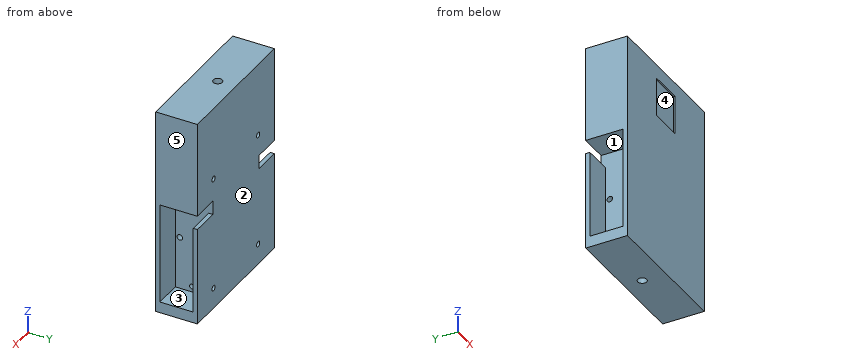
```python
from build123d import *

# Parameters (mm, degrees)
SKETCH1_W                    = 100
SKETCH1_H                    = 150
BOX_DEPTH                    = 30
SKETCH2_W                    = 73
SKETCH2_H                    = 24
MOTOR_COMPARTMENT_DEPTH      = 20
SKETCH3_W                    = 10
SKETCH3_H                    = 3
MOTOR_WIRE_PASSTHROUGH_DEPTH = 20
SKETCH4_R                    = 1.75
SKETCH4_R_2                  = 2
MOTOR_SCREW_MOUNT_DEPTH      = 10
SKETCH5_R                    = 2
MAKER_PI_MOUNT_HOLES_DEPTH   = 8
SKETCH6_W                    = 24
SKETCH6_H                    = 28
CASTER_MOUNT_DEPTH           = 1
SKETCH7_R                    = 3.2
FRONT_MOUNT_HOLE_DEPTH       = 25.4


with BuildPart() as part:
    # Sketch1 → box (new body)
    with BuildSketch(Plane(origin=(0, 0, 0), x_dir=(1, 0, 0), z_dir=(0, 1, 0))):
        Rectangle(SKETCH1_W, SKETCH1_H)
    extrude(amount=-BOX_DEPTH)

    # Sketch2 → motor compartment (cut)
    with BuildSketch(Plane(origin=(50, 0, 0), x_dir=(0, 0, -1), z_dir=(1, 0, 0))):
        with Locations((30.5, -15)):
            Rectangle(SKETCH2_W, SKETCH2_H)
    motor_compartment = extrude(amount=-MOTOR_COMPARTMENT_DEPTH, mode=Mode.SUBTRACT)

    # Sketch3 → motor wire passthrough (cut)
    with BuildSketch(Plane(origin=(50, 0, 0), x_dir=(0, 0, -1), z_dir=(1, 0, 0))):
        with Locations((-1, -1.5)):
            Rectangle(SKETCH3_W, SKETCH3_H)
    motor_wire_passthrough = extrude(amount=-MOTOR_WIRE_PASSTHROUGH_DEPTH, mode=Mode.SUBTRACT)

    # Sketch4 → motor screw mount (cut)
    with BuildSketch(Plane(origin=(30, 0, 0), x_dir=(0, 0, -1), z_dir=(1, 0, 0))):
        with Locations((63, -15)):
            Circle(SKETCH4_R)
        with Locations((28.75, -6.25)):
            Circle(SKETCH4_R_2)
        with Locations(Location((28.75, -23.75, 0), (0, 0, 180))):
            Circle(SKETCH4_R_2)
    motor_screw_mount = extrude(amount=-MOTOR_SCREW_MOUNT_DEPTH, mode=Mode.SUBTRACT)

    # motor compartment mirror: motor compartment, motor wire passthrough, motor screw mount across plane
    add(motor_compartment.mirror(Plane(origin=(0, 0, 0), x_dir=(0, 0, 1), z_dir=(1, 0, 0))), mode=Mode.SUBTRACT)
    add(motor_wire_passthrough.mirror(Plane(origin=(0, 0, 0), x_dir=(0, 0, 1), z_dir=(1, 0, 0))), mode=Mode.SUBTRACT)
    add(motor_screw_mount.mirror(Plane(origin=(0, 0, 0), x_dir=(0, 0, 1), z_dir=(1, 0, 0))), mode=Mode.SUBTRACT)

    # Sketch5 → Maker Pi mount holes (cut)
    with BuildSketch(Plane(origin=(0, 0, 0), x_dir=(1, 0, 0), z_dir=(0, 1, 0))):
        with Locations(Location((-29, 60, 0), (0, 0, 270))):
            Circle(SKETCH5_R)
        with Locations(Location((-29, -22, 0), (0, 0, 270))):
            Circle(SKETCH5_R)
        with Locations(Location((29, 60, 0), (0, 0, 300))):
            Circle(SKETCH5_R)
        with Locations(Location((29, -22, 0), (0, 0, 90))):
            Circle(SKETCH5_R)
    extrude(amount=-MAKER_PI_MOUNT_HOLES_DEPTH, mode=Mode.SUBTRACT)

    # Sketch6 → caster mount (cut)
    with BuildSketch(Plane.XZ.offset(30)):
        with Locations((0, 51)):
            Rectangle(SKETCH6_W, SKETCH6_H)
    extrude(amount=-CASTER_MOUNT_DEPTH, mode=Mode.SUBTRACT)

    # Sketch7 → front mount hole (cut)
    with BuildSketch(Plane.XY.offset(75)):
        with Locations((0, -13)):
            Circle(SKETCH7_R)
    front_mount_hole = extrude(amount=-FRONT_MOUNT_HOLE_DEPTH, mode=Mode.SUBTRACT)

    # back mount hole: front mount hole across plane
    add(front_mount_hole.mirror(Plane.XY), mode=Mode.SUBTRACT)


solid = part.part
```
Design review of the part built by this model. Coordinates are the model's own, in mm. Face numbers are marked on the shaded views. A direction names the side the tool comes from. Coordinates: 2 decimals unless noted, no trailing zeros. Order: outer loops, then holes, each group sorted by start corner. A loop starts at its lowest first (then second) coordinate and runs counter-clockwise, first axis right, second up. Notation, with made-up numbers: (71, -12) - (76, -12) arc R35 ccw to (76, 26) - close; hole circle Ø1 at (79.5, 77.5). An arc over 180 degrees is marked (long way). One line per question, with ' | ' between items.
Q1. Clearance check with flat-ended pins moving along their axes: pin 1 Ø1.2 at (x, z) = (-29, 21) entering from +Y; pin 2 Ø4 at (y, z) = (-15, -63) entering from -X; pin 3 Ø1.9 at (x, y) = (-0.5, -14) entering from -Z. State where each tip first meets the part, or that it passes through.
Answer key:
pin 1: stops at y = -8 | pin 2: stops at x = -30 | pin 3: stops at z = -49.6
Q2. The part is to be moulded in two halves that separate along X. For the marked faces 3, 4 and 5, say which applies: +X half, -X half, draft (parallel to the pull), parting line (faces both ways), or undercut.
Answer key:
face 3: draft | face 4: undercut | face 5: +X half
Q3. Consider section D-D, the plane z = -28.75. Give the boundary of the cut face in (x, y), then the cut area to 3 significant figures.
Answer key:
outline: (-50, -30) - (50, -30) - (50, -27) - (30, -27) - (30, -25.75) - (20, -25.75) - (20, -21.75) - (30, -21.75) - (30, -8.25) - (20, -8.25) - (20, -4.25) - (30, -4.25) - (30, -3) - (50, -3) - (50, 0) - (-50, 0) - (-50, -3) - (-30, -3) - (-30, -4.25) - (-20, -4.25) - (-20, -8.25) - (-30, -8.25) - (-30, -21.75) - (-20, -21.75) - (-20, -25.75) - (-30, -25.75) - (-30, -27) - (-50, -27) - close | area: 1,880 mm2
Q4. To check wall thickness, follow line 1 along Y through (x, z) = (-26.75, -28.75); line 2 along Z through (x, y) = (29, -3.25); line 3 along X through (y, z) = (-4, 22). State the ranges of each line that lie inside material, in increasing order.
Answer key:
line 1: y = -30 to -25.75, -21.75 to -8.25, -4.25 to 0 | line 2: z = -75 to -62, -58 to 20, 24 to 75 | line 3: x = -50 to -31, -27 to 27, 31 to 50
Q5. Consider section B-B, the plane z = -53. Give the boundary of the cut face in (x, y), then the cut area to 3 significant figures.
Answer key:
outline: (-50, -30) - (50, -30) - (50, -27) - (30, -27) - (30, -3) - (50, -3) - (50, 0) - (-50, 0) - (-50, -3) - (-30, -3) - (-30, -27) - (-50, -27) - close; hole circle Ø6.4 at (0, -13) | area: 2,010 mm2
Q6. For the marked faces 1 and 2, list the 3-axis set-ups (+Z, -Z, +X, -X, +Y, -Y) from which the entire face can be reached by the end or side of a thin tool; tool diameter is ignored.
Answer key:
face 1: -X, +Y | face 2: +Z, -Z, +X, -X, +Y
Q7. Consider section A-A, the plane z = -0.5. Give the boundary of the cut face in (x, y), then the cut area to 3 significant figures.
Answer key:
outline: (-50, -30) - (50, -30) - (50, -27) - (30, -27) - (30, 0) - (-30, 0) - (-30, -27) - (-50, -27) - close | area: 1,920 mm2
Q8. Consider section C-C, the plane x = 0. Give the boundary of the cut face in (y, z).
Answer key:
outline: (-30, -75) - (-16.2, -75) - (-16.2, -49.6) - (-9.8, -49.6) - (-9.8, -75) - (0, -75) - (0, 75) - (-9.8, 75) - (-9.8, 49.6) - (-16.2, 49.6) - (-16.2, 75) - (-30, 75) - (-30, 65) - (-29, 65) - (-29, 37) - (-30, 37) - close
